Autodesk Inventor part; units mm, degrees
ref_plane "YZ Plane" through (0, 0, 0) normal (1, 0, 0) x (0, 1, 0)
ref_plane "XZ Plane" through (0, 0, 0) normal (0, 1, 0) x (-1, 0, 0)
ref_plane "XY Plane" through (0, 0, 0) normal (0, 0, 1) x (1, 0, 0)
sketch "Sketch1" plane through (0, 0, 0) normal (0, 1, 0) x (-1, 0, 0)
  line L0 (0, 0) -> (22, 0)
  line L1 (22, 0) -> (22, -30)
  line L2 (22, -30) -> (0, -30)
  line L3 (0, -30) -> (0, 0)
  circle A0 centre (18.5, -26.5) radius 1.5
  circle A1 centre (3.5, -26.5) radius 1.5
  circle A2 centre (3.5, -3.5) radius 1.5
  circle A3 centre (18.5, -3.5) radius 1.5
  line L4 (11, -30) -> (11, 0)
  line L5 (22, -15) -> (0, -15)
  dimension "d0" = 30
  dimension "d1" = 22
  dimension "d3" = 3
  dimension "d34" = 15
  dimension "d35" = 23
  dimension "d36" = 23
  dimension "d37" = 15
extrude "Extrusion1" add sketch "Sketch1" along normal blind 1.5
sketch "Sketch2" plane through (0, 1.5, 0) normal (0, 1, 0) x (1, 0, 0)
  line L0 (-14.5, 27) -> (-7.5, 27)
  line L1 (-7.5, 27) -> (-7.5, 29)
  line L2 (-7.5, 29) -> (-14.5, 29)
  line L3 (-14.5, 29) -> (-14.5, 27)
  line L4 (0, 30) -> (-22, 30)
  line L5 (-22, 0) -> (0, 0)
  line L6 (-11, 0) -> (-11, 30)
  line L7 (-8, 6) -> (-14, 6)
  line L8 (-14, 6) -> (-14, 11)
  line L9 (-14, 11) -> (-8, 11)
  line L10 (-8, 11) -> (-8, 6)
  dimension "d14" = 7
  dimension "d15" = 2
  dimension "d16" = 1
  dimension "d20" = 5
  dimension "d21" = 6
  dimension "d22" = 6
extrude "Extrusion2" add sketch "Sketch2" along normal blind 8
sketch "Sketch3" plane through (-7.5, 1.5, -29) normal (0, 0, -1) x (-1, 0, 0)
  line L0 (0.5, 4) -> (6.5, 4)
  line L1 (6.5, 4) -> (6.5, 5)
  line L2 (6.5, 5) -> (0.5, 5)
  line L3 (0.5, 5) -> (0.5, 4)
  line L4 (-7.5, 0) -> (14.5, 0)
  line L5 (0, 0) -> (0, 8)
  line L6 (7, 0) -> (7, 8)
  point P0 (-7.5, -1.5)
  dimension "d25" = 4
  dimension "d26" = 6
  dimension "d27" = 1
  dimension "d28" = 0.5
  dimension "d29" = 0.5
extrude "Extrusion3" add sketch "Sketch3" along normal blind 8
sketch "Sketch4" plane through (-7.5, 1.5, -29) normal (0, 0, -1) x (-1, 0, 0)
  line L0 (6.5, 5) -> (0.5, 5)
  line L1 (6.5, 4) -> (0.5, 4)
  line L2 (0.5, 4) -> (0.5, 5)
  line L3 (0.5, 5) -> (6.5, 5)
  line L4 (6.5, 5) -> (6.5, 4)
  line L5 (7, 0) -> (0, 0)
  line L6 (7, 0) -> (7, 8)
  line L7 (0, 8) -> (7, 8)
  line L8 (0, 0) -> (0, 8)
  line L9 (0, 5) -> (7, 5)
  point P0 (-7.5, -1.5)
extrude "Extrusion4" cut sketch "Sketch4" against normal blind 8 contours L0 L9 L8 L7 L6
properties part number "IR_Receiver"
The listing builds one solid part. Answer for the finished solid, in the listing's coordinates (mm). A direction names the side the tool comes from. Coordinates: 2 decimals unless noted, no trailing zeros. Loops run counter-clockwise (first coordinate to the right, second up) from the corner with the lowest first, then second, coordinate; pieces in that order, holes last.
1) Find section C-C on y = 3.5. Write down the section's boundary in (x, z), then the cut area to 3 significant figures.
2) Find section B-B on x = -3.5. Write down the section's boundary in (y, z).
3) Find section A-A on z = -3.5. Write down the section's boundary in (x, y).
4) Flat-ended cylindrical pins translate along their axes: pin 1 Ø3.5 at (x, z) = (-18.5, -26.5) entering from +Y; pin 2 Ø2.5 at (y, z) = (5, -7.5) entering from +X; pin 3 Ø7.5 at (x, z) = (-10, -34) entering from +Y; pin 4 Ø10 at (x, z) = (-17.5, -27) entering from -Y. Find the tip coordinate at first contact, or state that the pin passes through.
5) A tool of negligible diameter and unlimited length cuts with its end or side. For faces 4 (the face through (-14, 5, -8)), 5 (the face through (-11, 5, -6)), 6 (the face through (-14.5, 4, -28)), 7 (the face through (-11, 4, -27)), 8 (the face through (-11, 1, -30)), from which of +Z, -Z, +X, -X, +Y, -Y can it reach the whole face along a straight path? Write none if from no direction.
6) Find section D-D on x = -9. Write down the section's boundary in (y, z), then the cut area to 3 significant figures.
7) Find the intervals of material crossed by L1, parallel to Z at x = -18.5, y = 1.1; L2, parallel to Y at x = -17, z = -13.5; L3, parallel to Z at x = -10.75, y = 3.75, in increasing order.
8) Determine the mould class of faces 1 (the face through (-11, 6.5, -32)), 2 (the face through (-3.305, 0.74, -27.987)), 3 (the face through (-11, 3, -29)) for opening direction Y: pulls with the +Y half, pulls with the -Y half, needs draft (parallel to the pull), parting line crosses it, or undercut.
Values:
1. outline: (-14.5, -29) - (-7.5, -29) - (-7.5, -27) - (-14.5, -27) - close; (-14, -11) - (-8, -11) - (-8, -6) - (-14, -6) - close
1. area: 44.0 mm2
2. outline: (0, -30) - (1.5, -30) - (1.5, -28) - (0, -28) - close; (0, -25) - (1.5, -25) - (1.5, -5) - (0, -5) - close; (0, -2) - (1.5, -2) - (1.5, 0) - (0, 0) - close
3. outline: (-22, 0) - (-20, 0) - (-20, 1.5) - (-22, 1.5) - close; (-17, 0) - (-5, 0) - (-5, 1.5) - (-17, 1.5) - close; (-2, 0) - (0, 0) - (0, 1.5) - (-2, 1.5) - close
4. pin 1: stops at y = 1.5
4. pin 2: stops at x = -8
4. pin 3: stops at y = 6.5
4. pin 4: stops at y = 0
5. face 4: +Z, -X, +Y
5. face 5: +Z, +X, -X, +Y
5. face 6: +Z, -Z, -X, +Y
5. face 7: +X, -X, +Y
5. face 8: -Z, +X, -X, -Y
6. outline: (0, -30) - (1.5, -30) - (1.5, -29) - (5.5, -29) - (5.5, -37) - (6.5, -37) - (6.5, -27) - (1.5, -27) - (1.5, -11) - (9.5, -11) - (9.5, -6) - (1.5, -6) - (1.5, 0) - (0, 0) - close
6. area: 103 mm2
7. L1: z = -30 to -28, -25 to -5, -2 to 0
7. L2: y = 0 to 1.5
7. L3: z = -29 to -27, -11 to -6
8. face 1: pulls with the +Y half
8. face 2: needs draft
8. face 3: undercut
